Answer from the drawing. Dimensions are ordinates in mm from the lowest x, y and z of the part. Coordinates: 2 decimals unless noted, no trailing zeros. Order: outer loops, then holes, each group sorted by start corner. A loop starts at its lowest first (then second) coordinate and runs counter-clockwise, first axis right, second up. Notation, with made-up numbers: (8.25, 87.5) -> (23.25, 87.5) arc R25 cw to (23.25, 126.5) -> close; hole circle Ø9 at (47.25, 70). An arc over 180 degrees is marked (long way). Use CSV: the item, a comma, the result in double quotes.
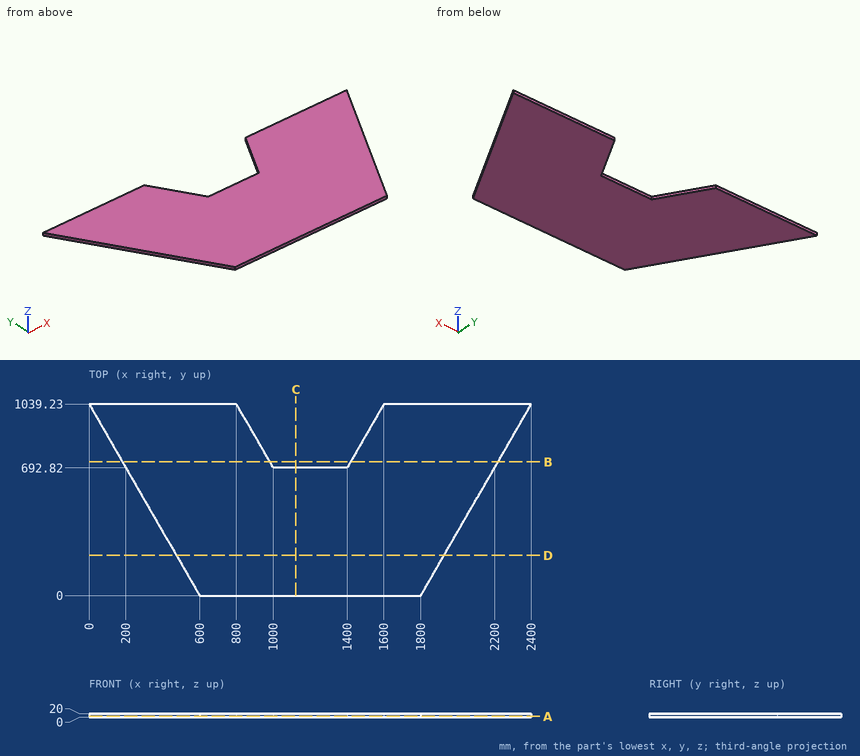
Item 1: Each of these flat-tipped pins is pushed along its axis until it touches: P1, Ø10, axis at x = 1172, z = 8, coming from the +Y side; P2, Ø6, axis at y = 902.5, z = 12.5, coming from the -X side; P3, Ø10, axis at y = 259.5, z = 11, coming from the +X side. Where does it stop, or does it pass through?
Return value:
P1,"stops at y = 692.82"
P2,"stops at x = 77.21"
P3,"stops at x = 1952.71"
Item 2: Find section A-A, the plane z = 4.5. Give the vertices of the cut face in (x, y), then the cut area to 3 significant figures.
Return value:
outline,"(0, 1039.23) -> (600, 0) -> (1800, 0) -> (2400, 1039.23) -> (1600, 1039.23) -> (1400, 692.82) -> (1000, 692.82) -> (800, 1039.23) -> close"
area,"1,660,000 mm^2"
Item 3: Find section C-C, the plane x = 1122. Give the vertices of the cut face in (y, z).
Return value:
outline,"(0, 0) -> (692.82, 0) -> (692.82, 20) -> (0, 20) -> close"
Item 4: Find section B-B, the plane y = 725.5. Give the vertices of the cut face in (x, z).
Return value:
outline,"(181.13, 0) -> (981.13, 0) -> (981.13, 20) -> (181.13, 20) -> close; (1418.87, 0) -> (2218.87, 0) -> (2218.87, 20) -> (1418.87, 20) -> close"
Item 5: Find section D-D, the plane y = 217.5. Give the vertices of the cut face in (x, z).
Return value:
outline,"(474.43, 0) -> (1925.57, 0) -> (1925.57, 20) -> (474.43, 20) -> close"
Item 6: Straight lines are drawn through the part: line 1 along X through (y, z) = (866, 19) (1 decimal); line 2 along X through (y, z) = (824.5, 10.5) (1 decimal); line 3 along Y through (x, z) = (2117, 3.75). For each, find the intervals that lie inside material, in ascending order.
Return value:
line 1,"x = 100 to 900, 1500 to 2300"
line 2,"x = 124 to 924, 1476 to 2276"
line 3,"y = 549.06 to 1039.23"
